Autodesk Inventor part; units mm, degrees
ref_plane "工作平面1" through (10, 22, 0) normal (-0.3682, -0.6574, -0.6574) x (0.8725, 0, -0.4886)
ref_plane "YZ Plane" through (0, 0, 0) normal (1, 0, 0) x (0, 1, 0)
ref_plane "XZ Plane" through (0, 0, 0) normal (0, 1, 0) x (-1, 0, 0)
sketch "草圖1" plane through (0, 0, 0) normal (0, 1, 0) x (-1, 0, 0)
  line L0 (0, 0) -> (-60, 0)
  line L1 (-60, 0) -> (-60, -38)
  line L2 (-60, -38) -> (0, -38)
  line L3 (0, -38) -> (0, 0)
  dimension "d0" = 60
  dimension "d1" = 38
extrude "擠出1" add sketch "草圖1" along normal mid plane 44
sketch "草圖2" plane through (0, 22, 0) normal (0, 1, 0) x (1, 0, 0)
  line L0 (0, 0) -> (60, 0)
  line L1 (10, 0) -> (60, 8)
  line L2 (60, 0) -> (60, 38)
  dimension "d4" = 10
  dimension "d5" = 30
extrude "擠出2" cut sketch "草圖2" against normal blind 60
sketch "草圖3" plane through (60, -22, -38) normal (1, 0, 0) x (0, 0, -1)
  line L0 (-30, 24) -> (-10, 44)
  line L1 (0, 44) -> (-38, 44)
  line L2 (-30, 44) -> (-30, 0)
  point P0 (-38, 22)
  point P1 (-30, 2)
  dimension "d8" = 20
  dimension "d9" = 20
ref_plane "工作平面1" through (10, 22, 0) normal (-0.3682, -0.6574, -0.6574) x (0.8725, 0, -0.4886)
sketch "草圖4" plane through (10, 22, 0) normal (-0.3682, -0.6574, -0.6574) x (0.8725, 0, -0.4886)
  line L0 (-15.1543, -12.3218) -> (93.717, -12.3218)
  line L1 (93.717, -12.3218) -> (93.717, 28.8166)
  line L2 (93.717, 28.8166) -> (-15.1543, 28.8166)
  line L3 (-15.1543, 28.8166) -> (-15.1543, -12.3218)
  point P0 (-8.7251, 13.3649)
extrude "擠出3" cut sketch "草圖4" against normal blind 40
mirror "鏡射1" about plane through (0, 0, 0) normal (0, 1, 0) of "擠出3"
properties part number "53"
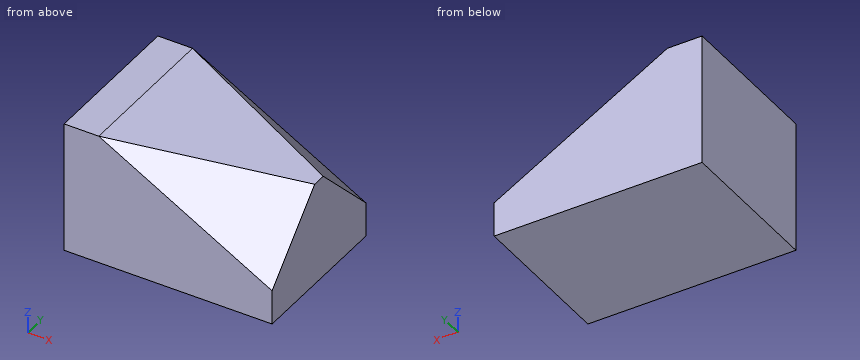
The listing builds one solid part. Answer for the finished solid, in the listing's coordinates (mm). Give positions to 0.01 mm unless a question says otherwise; leave off trailing zeros. Order: outer loops, then holes, each group sorted by start corner. A loop starts at its lowest first (then second) coordinate and runs counter-clockwise, first axis right, second up. Notation, with made-up numbers: (89.25, 13.5) -> (142.25, 13.5) arc R21 ccw to (142.25, 46.5) -> close; hole circle Ø2 at (79.25, 65). An arc over 180 degrees is marked (long way). One line per item, written item: value.
1) Find the intervals of material crossed by line 1 (X direction, y = -7.5, z = -10); line 2 (X direction, y = 17, z = -2.5); line 3 (Z direction, x = 22.5, y = 13), in increasing order.
Reported:
line 1: x = 0 to 53.74
line 2: x = 0 to 23.39
line 3: z = -38 to -2
2) Find section B-B, the plane y = -19. Determine the outline of the cut face in (x, z).
Reported:
outline: (0, -38) -> (60, -38) -> (60, -25.01) -> (17.49, -1.2) -> (10, 0) -> (0, 0) -> close
3) Find section A-A, the plane z = -13. Determine the outline of the cut face in (x, y).
Reported:
outline: (0, -22) -> (33.21, -22) -> (60, -6.99) -> (60, 6.99) -> (33.21, 22) -> (0, 22) -> close
